```python
from build123d import *

# Parameters (mm, degrees)
SKETCH1_W               = 17
SKETCH1_H               = 30
BOSS_EXTRUDE1_DEPTH     = 1.5
SKETCH2_W               = 11
SKETCH2_H               = 3
BOSS_EXTRUDE2_DEPTH     = 1.5
CUT_EXTRUDE1_DEPTH      = 20.962464778
CUT_EXTRUDE1_DEPTH_BACK = 20.962464778
SKETCH3_W               = 5
SKETCH3_H               = 3
CUT_EXTRUDE2_DEPTH      = 20.962464778
CUT_EXTRUDE2_DEPTH_BACK = 20.962464778


with BuildPart() as part:
    # Sketch1 → Boss-Extrude1 (new, symmetric)
    with BuildSketch(Plane(origin=(0, 0, 0), x_dir=(1, 0, 0), z_dir=(0, 1, 0))):
        Rectangle(SKETCH1_W, SKETCH1_H)
    extrude(amount=BOSS_EXTRUDE1_DEPTH, both=True)

    # Sketch2 → Boss-Extrude2 (add, symmetric)
    with BuildSketch(Plane(origin=(0, 0, 0), x_dir=(1, 0, 0), z_dir=(0, 1, 0))):
        with Locations((0, -16.5)):
            Rectangle(SKETCH2_W, SKETCH2_H)
    extrude(amount=BOSS_EXTRUDE2_DEPTH, both=True)

    # Sketch3 → Cut-Extrude1 (cut, two sides: drawn at the far end of the back side and taken through both)
    with BuildSketch(Plane(origin=(0, 0, 0), x_dir=(1, 0, 0), z_dir=(0, 1, 0)).offset(-CUT_EXTRUDE1_DEPTH_BACK)):
        with Locations((0, -3.5)):
            Rectangle(SKETCH3_W, SKETCH3_H)
    extrude(amount=CUT_EXTRUDE1_DEPTH + CUT_EXTRUDE1_DEPTH_BACK, mode=Mode.SUBTRACT)

    # Sketch4 → Cut-Extrude2 (cut, two sides: drawn at the far end of the back side and taken through both)
    with BuildSketch(Plane(origin=(0, 0, 0), x_dir=(1, 0, 0), z_dir=(0, 1, 0)).offset(-CUT_EXTRUDE2_DEPTH_BACK)):
        with BuildLine():
            Line((-1.5, -18), (1.5, -18))
            Line((1.5, -18), (1.5, -14))
            Line((1.5, -14), (2.85, -14))
            Line((2.85, -14), (2.85, -11.73))
            Line((2.85, -11.73), (1.5, -11.73))
            Line((1.5, -11.73), (1.5, -9))
            ThreePointArc((1.5, -9), (1.207106781, -8.292893219), (0.5, -8))
            Line((0.5, -8), (-0.5, -8))
            ThreePointArc((-0.5, -8), (-1.207106781, -8.292893219), (-1.5, -9))
            Line((-1.5, -9), (-1.5, -11.73))
            Line((-1.5, -11.73), (-2.85, -11.73))
            Line((-2.85, -11.73), (-2.85, -14))
            Line((-2.85, -14), (-1.5, -14))
            Line((-1.5, -14), (-1.5, -18))
        make_face()
    extrude(amount=CUT_EXTRUDE2_DEPTH + CUT_EXTRUDE2_DEPTH_BACK, mode=Mode.SUBTRACT)


solid = part.part
```
CAD build for the part. Positions are in the model's coordinates, mm. A direction names the side the tool comes from. Give positions to 0.01 mm unless a question says otherwise; leave off trailing zeros. Loops run counter-clockwise (first coordinate to the right, second up) from the corner with the lowest first, then second, coordinate; pieces in that order, holes last. Notation, with made-up numbers: (8.25, -33.5) - (53.25, -33.5) arc R17 ccw to (53.25, -9.5) - close; hole circle Ø1 at (-18, -39). An arc over 180 degrees is marked (long way). Put each result on its own line as item: value.
Q1. Probe line 1 along Z through (x, y) = (1.75, 0.55); line 2 along X through (y, z) = (0.3, 3); line 3 along X through (y, z) = (0.85, 13). List the from-to ranges inside material, lowest first.
Filled in:
line 1: z = -15 to 2, 5 to 11.73, 14 to 18
line 2: x = -8.5 to -2.5, 2.5 to 8.5
line 3: x = -8.5 to -2.85, 2.85 to 8.5
Q2. Slice it at B-B (y = 0). Give the cut face in (x, z), plus the area to 3 significant figures.
Filled in:
outline: (-8.5, -15) - (8.5, -15) - (8.5, 15) - (5.5, 15) - (5.5, 18) - (1.5, 18) - (1.5, 14) - (2.85, 14) - (2.85, 11.73) - (1.5, 11.73) - (1.5, 9) arc R1 cw to (0.5, 8) - (-0.5, 8) arc R1 cw to (-1.5, 9) - (-1.5, 11.73) - (-2.85, 11.73) - (-2.85, 14) - (-1.5, 14) - (-1.5, 18) - (-5.5, 18) - (-5.5, 15) - (-8.5, 15) - close; hole (-2.5, 2) - (2.5, 2) - (2.5, 5) - (-2.5, 5) - close
area: 492 mm²
Q3. Slice it at A-A (z = 13.5). Give the cut face in (x, y), plus the area to 3 significant figures.
Filled in:
outline: (-8.5, -1.5) - (-2.85, -1.5) - (-2.85, 1.5) - (-8.5, 1.5) - close; (2.85, -1.5) - (8.5, -1.5) - (8.5, 1.5) - (2.85, 1.5) - close
area: 33.9 mm²
Q4. Flat gauge pins, fed straight in: pin 1 (1.1 mm diameter, centred on x = 0, y = 0.5, fed in from +Z); pin 2 (0.9 mm diameter, centred on y = 0.5, z = 17, fed in from +X); pin 3 (1.5 mm diameter, centred on x = -7.5, y = -0.5, fed in from +Z). Where does each tip first touch, or does it go through?
Filled in:
pin 1: stops at z = 8
pin 2: stops at x = 5.5
pin 3: stops at z = 15
Q5. Slice it at C-C (z = 3). Give the cut face in (x, y), plus the area to 3 significant figures.
Filled in:
outline: (-8.5, -1.5) - (-2.5, -1.5) - (-2.5, 1.5) - (-8.5, 1.5) - close; (2.5, -1.5) - (8.5, -1.5) - (8.5, 1.5) - (2.5, 1.5) - close
area: 36.0 mm²
Q6. Slice it at D-D (x = 6.25). Give the cut face in (y, z), plus the area to 3 significant figures.
Filled in:
outline: (-1.5, -15) - (1.5, -15) - (1.5, 15) - (-1.5, 15) - close
area: 90.0 mm²
Q7. Tool access for faces 1 (the face through (-7, 0, 15)), 2 (the face through (5.5, 0, 17)), 3 (the face through (1.215, -0.021, 8.301)), 4 (the face through (2, 0, 14)): list every direction of +Z, -Z, +X, -X, +Y, -Y with a clear straight run to the whole face (end or side of a thin tool).
Filled in:
face 1: +Z, -X, +Y, -Y
face 2: +Z, +X, +Y, -Y
face 3: +Z, +Y, -Y
face 4: +Y, -Y
Q8. Mould opens along X. For faces 5 (the face through (1.5, 0, 10)), 6 (the face through (-4, 0, 18)), 7 (the face through (-1.5, 0, 10)), 8 (the face through (-5.5, 0, 17)) say: pulls with the +X half, pulls with the -X half, needs draft (parallel to the pull), parting line crosses it, or undercut.
Filled in:
face 5: undercut
face 6: needs draft
face 7: undercut
face 8: pulls with the -X half
